For this review, take the finished solid that the model builds, in its own axes (mm). A direction names the side the tool comes from. Round coordinates to 2 decimals unless told otherwise and drop trailing zeros. Order: outer loops, then holes, each group sorted by start corner. A loop starts at its lowest first (then second) coordinate and runs counter-clockwise, first axis right, second up. Notation, with made-up numbers: (-39, -34.75) -> (-8, -34.75) arc R28 ccw to (-8, -1.75) -> close; hole circle Ø1 at (-34, 10.5). An arc over 180 degrees is marked (long way). Use a Markdown table: item, result. Add a question column.
1) Draft analysis for pull direction Z (two halves, no side actions). For faces 5 (the face through (164.465, -241, -250)), 6 (the face through (-159.385, -254, 368)), 7 (the face through (-191, -242, -508)), 8 (the face through (158.115, -254, 190)), state which applies: pulls with the +Z half, pulls with the -Z half, needs draft (parallel to the pull), parting line crosses it, or undercut.
2) Consider section C-C (z = -199). State the section outline as (x, y) points (3 decimals), plus the area to 3 significant figures.
3) Consider section B-B (x = 181.5). State the section outline as (y, z) points, plus the area to 3 significant figures.
4) Wall thickness on line 1 along Y through (x, z) = (-181, -42); line 2 along Y through (x, z) = (165.5, -187); line 3 along X through (y, z) = (172.5, -86.5) (3 decimals): over which ranges is each line inside the solid? List them lowest first. Write a range as [from, to].
5) Consider section A-A (z = 274.5). State the section outline as (x, y) points (3 decimals).
6) Clearance check with flat-ended pins moving along their axes: P1, Ø4, axis at x = -98, y = -30, coming from the +Z side; P2, Ø15, axis at x = 41, y = -256, coming from the -Z side; P3, Ø8, axis at x = 165, z = 124, coming from the +Y side. State where each tip first meets the part, or that it passes through.
7) Consider section D-D (z = -29). State the section outline as (x, y) points (3 decimals), plus the area to 3 significant figures.
8) Machinability: for faces 1 (the face through (222.236, 4.195, 70.768)), 2 (the face through (190, -215.9, -250)), 3 (the face through (-143, -50, 76.2)), 4 (the face through (-216.535, 174, -250)), which of the approach directions +Z, -Z, +X, -X, +Y, -Y give a long, thin tool a straight path to every point of the face, cutting with its end or side? Answer none if there is none.
```python
from build123d import *

# Parameters (mm, degrees)
F2_W      = 457.2
F2_H      = 457.2
F3_DEPTH  = 50.8
F0_W      = 457.2
F0_H      = 457.2
F4_DEPTH  = 76.2
F5_W      = 50.8
F5_H      = 50.8
F6_DEPTH  = 508
F7_R      = 19.05
F8_W      = 317.5
F8_H      = 38.1
F9_DEPTH  = 63.5
F10_R     = 31.7295136587
F10_R_2   = 22.617106641
F11_DEPTH = 63.5
F12_R     = 147.0598184699
F13_DEPTH = 2.54
F15_R     = 5.08
F16_R     = 5.08


# Not quite as in the source:
# - a fillet or chamfer that OpenCascade refuses, or shapes differently, is made with other operations: its cross-section is extruded or revolved along the edge and cut away or added


with BuildPart() as f3:
    # F2 (on offset) → F3 (new body)
    with BuildSketch(Plane.XZ.offset(228.6)):
        with Locations((-0.6349999458, 228.6)):
            Rectangle(F2_W, F2_H)
    extrude(amount=F3_DEPTH)

    # F0 (on Top) → F4 (join)
    with BuildSketch(Plane.XY):
        with Locations((-0.6349999458, -16.5623649633)):
            Rectangle(F0_W, F0_H)
    extrude(amount=F4_DEPTH)

    # F5 (on face) → F6 (join)
    with BuildSketch(Plane(origin=(0, 0, 0), x_dir=(1, 0, 0), z_dir=(0, 0, -1))):
        with Locations((-191.1349999458, 241.3)):
            Rectangle(F5_W, F5_H)
        with Locations((189.8650000542, 241.3)):
            Rectangle(F5_W, F5_H)
        with Locations((189.8650000542, -173.9376350367)):
            Rectangle(F5_W, F5_H)
        with Locations((-191.1349999458, -173.9376350367)):
            Rectangle(F5_W, F5_H)
    extrude(amount=F6_DEPTH)

    # F7
    f7_edges = [f3.edges().sort_by_distance(p)[0] for p in [
        (-0.635, -228.6, 76.2),
        (-0.635, -228.6, 457.2),
        (-229.235, -228.6, 266.7),
        (227.965, -228.6, 266.7),
        (-0.635, -279.4, 457.2),
        (227.965, -279.4, 228.6),
        (227.965, -254, 457.2),
        (-229.235, -254, 457.2),
        (-229.235, -8.281182, 76.2),
        (227.965, -8.281182, 76.2),
        (-0.635, 212.037635, 76.2),
        (-229.235, -279.4, 228.6),
    ]]
    fillet(f7_edges, radius=F7_R)

    # F8 (on face) → F9 (cut, symmetric)
    with BuildSketch(Plane.XZ.offset(279.4)):
        with Locations((-0.6349999458, 368.3)):
            Rectangle(F8_W, F8_H)
        with Locations((-0.6349999458, 279.4)):
            Rectangle(F8_W, F8_H)
        with Locations((-0.6349999458, 190.5)):
            Rectangle(F8_W, F8_H)
    extrude(amount=F9_DEPTH, both=True, mode=Mode.SUBTRACT)

    # F10 (on face) → F11 (join)
    with BuildSketch(Plane(origin=(0, 0, 0), x_dir=(1, 0, 0), z_dir=(0, 0, -1))):
        with Locations((-183.2177340984, 168.4852540493)):
            Circle(F10_R)
        with Locations((-183.2177340984, 168.4852540493)):
            Circle(F10_R_2, mode=Mode.SUBTRACT)
    extrude(amount=F11_DEPTH)

    # F12 (on face) → F13 (cut)
    with BuildSketch(Plane.XY.offset(76.2)):
        Circle(F12_R)
    extrude(amount=-F13_DEPTH, mode=Mode.SUBTRACT)

    # F14: fillet of radius 5.08 on 1 edges, made by hand

    # F14_s1 → F14_t2 (revolve)
    with BuildSketch(Plane.XZ):
        with BuildLine():
            ThreePointArc((147.0598184699, 76.2), (145.2004094187, 74.3405909488), (142.6604094187, 73.66))
            Line((142.6604094187, 73.66), (147.0598184699, 73.66))
            Line((147.0598184699, 73.66), (147.0598184699, 76.2))
        make_face()
    revolve(axis=Axis((0, 0, 73.66), (0, 0, 1)))

    # F15
    f15_edges = [f3.edges().sort_by_distance(p)[0] for p in [
        (-147.059818, 0, 76.2),
    ]]
    fillet(f15_edges, radius=F15_R)

    # F16
    f16_edges = [f3.edges().sort_by_distance(p)[0] for p in [
        (-229.235, -24.156182, 0),
        (-0.635, 212.037635, 0),
        (227.965, -24.156182, 0),
        (-0.635, -279.4, 0),
        (222.385384, -273.820384, 0),
        (-223.655384, -273.820384, 0),
    ]]
    fillet(f16_edges, radius=F16_R)


solid = f3.part
```
Results list:
| question | item | result |
|---|---|---|
| 1 | face 5 | needs draft |
| 1 | face 6 | undercut |
| 1 | face 7 | pulls with the -Z half |
| 1 | face 8 | undercut |
| 2 | outline | (-216.535, -266.7) -> (-165.735, -266.7) -> (-165.735, -215.9) -> (-216.535, -215.9) -> close; (-216.535, 148.538) -> (-165.735, 148.538) -> (-165.735, 199.338) -> (-216.535, 199.338) -> close; (164.465, -266.7) -> (215.265, -266.7) -> (215.265, -215.9) -> (164.465, -215.9) -> close; (164.465, 148.538) -> (215.265, 148.538) -> (215.265, 199.338) -> (164.465, 199.338) -> close |
| 2 | area | 10,300 mm2 |
| 3 | outline | (-279.4, 5.08) arc R5.08 ccw to (-274.32, 0) -> (-266.7, 0) -> (-266.7, -508) -> (-215.9, -508) -> (-215.9, 0) -> (148.54, 0) -> (148.54, -508) -> (199.34, -508) -> (199.34, 0) -> (206.96, 0) arc R5.08 ccw to (212.04, 5.08) -> (212.04, 57.15) arc R19.05 ccw to (192.99, 76.2) -> (-209.55, 76.2) arc R19.05 cw to (-228.6, 95.25) -> (-228.6, 438.15) arc R19.05 ccw to (-247.65, 457.2) -> (-260.35, 457.2) arc R19.05 ccw to (-279.4, 438.15) -> close |
| 3 | area | 108,000 mm2 |
| 4 | line 1 | [-266.7, -215.9], [-200.14, -190.99], [-145.98, -136.83], [148.54, 199.34] |
| 4 | line 2 | [-266.7, -215.9], [148.54, 199.34] |
| 4 | line 3 | [-216.535, -165.735], [164.465, 215.265] |
| 5 | outline | (-229.235, -260.35) arc R19.05 ccw to (-210.185, -279.4) -> (-159.385, -279.4) -> (-159.385, -228.6) -> (-210.185, -228.6) arc R19.05 ccw to (-229.235, -247.65) -> close; (158.115, -279.4) -> (208.915, -279.4) arc R19.05 ccw to (227.965, -260.35) -> (227.965, -247.65) arc R19.05 ccw to (208.915, -228.6) -> (158.115, -228.6) -> close |
| 6 | P1 | z = 73.66 |
| 6 | P2 | z = 0 |
| 6 | P3 | y = -228.6 |
| 7 | outline | (-216.535, -266.7) -> (-165.735, -266.7) -> (-165.735, -215.9) -> (-216.535, -215.9) -> close; (-216.535, 148.538) -> (-165.735, 148.538) -> (-165.735, 199.338) -> (-216.535, 199.338) -> close; circle Ø63.459 at (-183.218, -168.485); (164.465, -266.7) -> (215.265, -266.7) -> (215.265, -215.9) -> (164.465, -215.9) -> close; (164.465, 148.538) -> (215.265, 148.538) -> (215.265, 199.338) -> (164.465, 199.338) -> close; hole circle Ø45.234 at (-183.218, -168.485) |
| 7 | area | 11,900 mm2 |
| 8 | face 1 | +Z, +X, +Y |
| 8 | face 2 | -Z, +X, -X |
| 8 | face 3 | +Z, +X, -X, +Y |
| 8 | face 4 | -Z, -X, +Y, -Y |
